Autodesk Inventor part; units mm, degrees
ref_plane "YZ Plane" through (0, 0, 0) normal (1, 0, 0) x (0, 1, 0)
ref_plane "XZ Plane" through (0, 0, 0) normal (0, 1, 0) x (-1, 0, 0)
ref_plane "XY Plane" through (0, 0, 0) normal (0, 0, 1) x (1, 0, 0)
sketch "Sketch6" plane through (0, 0, 0) normal (1, 0, 0) x (0, 1, 0)
  line L0 (-50, 59.5) -> (50, 59.5)
  line L1 (50, 59.5) -> (50, -59.5)
  line L2 (50, -59.5) -> (-50, -59.5)
  line L3 (-50, -59.5) -> (-50, 59.5)
  line L4 (-50, 59.5) -> (50, -59.5) construction
  line L5 (50, 59.5) -> (-50, -59.5) construction
  point P0 (0, 0)
  dimension "d28" = 100
  dimension "d29" = 119
extrude "Extrusion5" add sketch "Sketch6" along normal mid plane 12
sketch "Sketch7" plane through (6, 0, 0) normal (1, 0, 0) x (0, 0, -1)
  line L0 (-59.5, 50) -> (-59.5, -50)
  line L1 (-59.5, -50) -> (-47.5, -50)
  line L2 (-47.5, -50) -> (-47.5, -30)
  line L3 (-47.5, -30) -> (-59.5, -30)
  line L4 (-59.5, -30) -> (-59.5, -50)
  line L5 (-59.5, -50) -> (-59.5, 50)
  line L6 (-59.5, -10) -> (-47.5, -10)
  line L7 (-47.5, -10) -> (-47.5, 10)
  line L8 (-47.5, 10) -> (-59.5, 10)
  line L9 (-59.5, 10) -> (-59.5, -10)
  line L10 (-59.5, 30) -> (-47.5, 30)
  line L11 (-47.5, 30) -> (-47.5, 50)
  line L12 (-47.5, 50) -> (-59.5, 50)
  line L13 (-59.5, 50) -> (-59.5, 30)
  point P0 (0, 0)
  dimension "d32" = 12
  dimension "d33" = 20
  dimension "d34" = 12
  dimension "d35" = 20
  dimension "d36" = 20
  dimension "d39" = 12
  dimension "d40" = 20
  dimension "d41" = 20
extrude "Extrusion6" cut sketch "Sketch7" against normal through all
mirror "Mirror2" about plane through (0, 0, 0) normal (0, 0, 1) of "Extrusion6"
sketch "Sketch8" plane through (6, 0, 0) normal (1, 0, 0) x (0, 0, -1)
  circle A0 centre (0, 0) radius 5
  dimension "d44" = 10
extrude "Extrusion7" cut sketch "Sketch8" against normal through all
properties part number "FRONT V2" material "Wood (Cherry)"
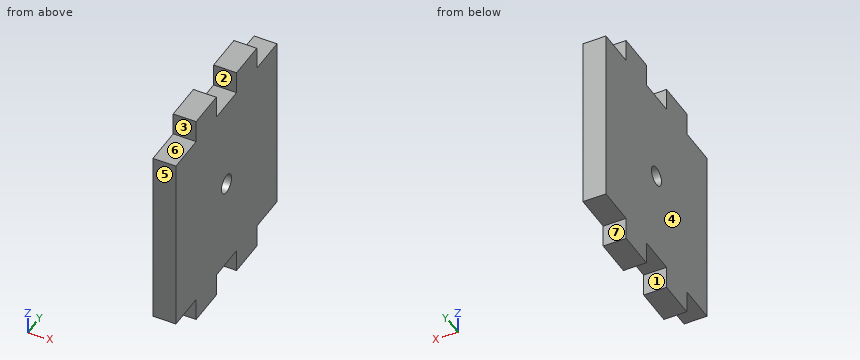
Source: CAD feature listing. Evaluate the final solid. Frame: model axes, mm. Face numbers are marked on the shaded views. A direction names the side the tool comes from. Round coordinates to 2 decimals unless told otherwise and drop trailing zeros. Order: outer loops, then holes, each group sorted by start corner. A loop starts at its lowest first (then second) coordinate and runs counter-clockwise, first axis right, second up. Notation, with made-up numbers: (11, 9) -> (45, 9) arc R22 cw to (45, 18) -> close; hole circle Ø5 at (-2, 82.5). An arc over 180 degrees is marked (long way). Answer as CSV lines item,"result".
Item 1: Section B-B, the plane z = 0. Return loops of the section in (x, y).
A:
outline,"(-6, -50) -> (6, -50) -> (6, -5) -> (-6, -5) -> close; (-6, 5) -> (6, 5) -> (6, 50) -> (-6, 50) -> close"
Item 2: Line query: L1, parallel to Y at x = -2.25, z = 0; L2, parallel to Z at x = 1.5, y = -34; L3, parallel to Z at x = -4, y = 2. Output: solid intervals per line, ascending.
A:
L1,"-50 to -5, 5 to 50"
L2,"-47.5 to 47.5"
L3,"-47.5 to -4.58, 4.58 to 47.5"
Item 3: Section A-A, the plane y = 0. Return loops of the section in (x, z), plus the area to 3 significant figures.
A:
outline,"(-6, -47.5) -> (6, -47.5) -> (6, -5) -> (-6, -5) -> close; (-6, 5) -> (6, 5) -> (6, 47.5) -> (-6, 47.5) -> close"
area,"1,020 mm²"
Item 4: Section C-C, the plane x = -3.5. Return loops of the section in (y, z), plus the area to 3 significant figures.
A:
outline,"(-50, -47.5) -> (-30, -47.5) -> (-30, -59.5) -> (-10, -59.5) -> (-10, -47.5) -> (10, -47.5) -> (10, -59.5) -> (30, -59.5) -> (30, -47.5) -> (50, -47.5) -> (50, 47.5) -> (30, 47.5) -> (30, 59.5) -> (10, 59.5) -> (10, 47.5) -> (-10, 47.5) -> (-10, 59.5) -> (-30, 59.5) -> (-30, 47.5) -> (-50, 47.5) -> close; hole circle Ø10 at (0, 0)"
area,"10,400 mm²"
Item 5: Pin query (flat end, axial travel): pin 1 Ø3.5 at (x, y) = (-0.5, 43.5) entering from +Z; pin 2 Ø3.5 at (x, z) = (-1.5, 54) entering from +Y; pin 3 Ø3.5 at (x, z) = (-2, 54.5) entering from -Y. Return the tip coordinate at first contact, or that it passes through.
A:
pin 1,"z = 47.5"
pin 2,"y = 30"
pin 3,"y = -30"
Item 6: Section D-D, the plane y = -32. Return loops of the section in (x, z), plus the area to 3 significant figures.
A:
outline,"(-6, -47.5) -> (6, -47.5) -> (6, 47.5) -> (-6, 47.5) -> close"
area,"1,140 mm²"
Item 7: Pull-direction query (Y, two-part tool) for the marked faces 1, 2, 3 and 4; classes: pulls with the +Y half, pulls with the -Y half, needs draft (parallel to the pull), parting line crosses it, or undercut.
A:
face 1,"undercut"
face 2,"undercut"
face 3,"pulls with the -Y half"
face 4,"needs draft"
Item 8: Reachability of the marked faces 5, 6 and 7 from +Z, -Z, +X, -X, +Y, -Y: full face, straight path, thin tool, end or side. Return the list, or none.
A:
face 5,"+Z, -Z, +X, -X, -Y"
face 6,"+Z, +X, -X, -Y"
face 7,"-Z, +X, -X, +Y"
